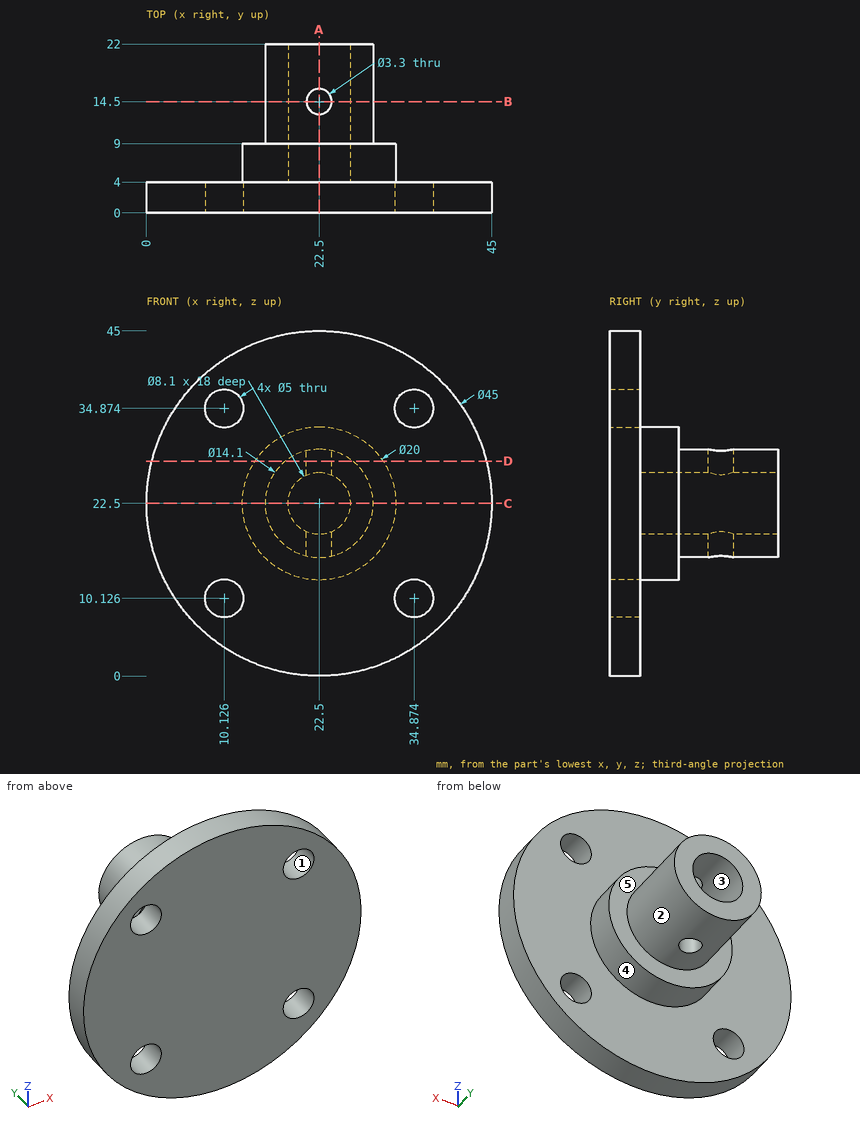
Part print with two shaded views. Sizes in mm from the minimum x, y, z corner. A direction names the side the tool comes from. Give positions to 0.01 mm unless a question says otherwise; leave off trailing zeros. Order: outer loops, then holes, each group sorted by start corner. A loop starts at its lowest first (then second) coordinate and runs counter-clockwise, first axis right, second up. Notation, with made-up numbers: M 89.5,89 L 126.5,89 A23 cw 126.5,120 Z; hole C 38.5,9.5 d4. An arc over 180 degrees is marked long. Write item = value, one per line.
Q1. Two-plate mould, pull along Z, no slides. Class the marked faces 3, 4 and 5: pulls with the +Z half, pulls with the -Z half, needs draft (parallel to the pull), parting line crosses it, or undercut.
Derived:
face_3 = undercut
face_4 = parting line crosses it
face_5 = needs draft
Q2. Cut at B-B, the plane y = 14.5. List the corners of the cut face in (x, z).
Derived:
outline = M 20.85,15.65 L 20.85,18.8 A4.05 cw 20.85,26.2 L 20.85,29.35 A7.05 ccw Z; M 24.15,15.65 A7.05 ccw 24.15,29.35 L 24.15,26.2 A4.05 cw 24.15,18.8 Z
Q3. Cut at C-C, the plane z = 22.5. List the corners of the cut face in (x, y).
Derived:
outline = M 0,0 L 45,0 L 45,4 L 32.5,4 L 32.5,9 L 29.55,9 L 29.55,22 L 26.55,22 L 26.55,4 L 18.45,4 L 18.45,22 L 15.45,22 L 15.45,9 L 12.5,9 L 12.5,4 L 0,4 Z
Q4. Tool access for the marked faces 1 and 2: list every direction of +Z, -Z, +X, -X, +Y, -Y with a clear straight run to the whole face (end or side of a thin tool).
Derived:
face_1 = +Y, -Y
face_2 = +Y
Q5. Flat gauge pins, fed straight in: pin 1 (6 mm diameter, centred on x = 24.5, z = 11.5, fed in from +Y); pin 2 (5.5 mm diameter, centred on x = 22.5, y = 14.5, fed in from +Z); pin 3 (4 mm diameter, centred on y = 3.5, z = 37.5, fed in from +X) (1 decimal). Where does each tip first touch, or does it go through?
Derived:
pin_1 = 9
pin_2 = 29.55
pin_3 = 40.9
Q6. Drill centre lines: line 1 (X direction, y = 17, z = 22.5); line 2 (Y direction, x = 22.5, z = 27.3). Where is each one in solid material? Low to high. Write a range as [from, to].
Derived:
line_1 = [15.45, 18.45], [26.55, 29.55]
line_2 = [0, 12.85], [16.15, 22]
Q7. Cut at A-A, the plane x = 22.5. List the corners of the cut face in (y, z).
Derived:
outline = M 0,0 L 4,0 L 4,12.5 L 9,12.5 L 9,15.45 L 12.85,15.45 L 12.85,18.45 L 4,18.45 L 4,26.55 L 12.85,26.55 L 12.85,29.55 L 9,29.55 L 9,32.5 L 4,32.5 L 4,45 L 0,45 Z; M 16.15,15.45 L 22,15.45 L 22,18.45 L 16.15,18.45 Z; M 16.15,26.55 L 22,26.55 L 22,29.55 L 16.15,29.55 Z
Q8. Cut at D-D, the plane z = 28. List the corners of the cut face in (x, y).
Derived:
outline = M 0.68,0 L 44.32,0 L 44.32,4 L 30.85,4 L 30.85,9 L 26.91,9 L 26.91,22 L 18.09,22 L 18.09,9 L 14.15,9 L 14.15,4 L 0.68,4 Z; hole C 22.5,14.5 d3.3
